Check sheet for the drawn part. Datum: minimum x, y, z corner. Units: mm. A direction names the side the tool comes from. Coordinates: 2 decimals unless noted, no trailing zeros. Loops run counter-clockwise (first coordinate to the right, second up) from the corner with the lowest first, then second, coordinate; pieces in that order, holes last. Notation, with made-up numbers: M -34.75,65.25 L 8.25,65.25 A30 cw 8.25,94.25 Z; hole C -12.5,-14 d4. An arc over 180 degrees is marked long. Answer in a Markdown table with one row per item. Add a question column.
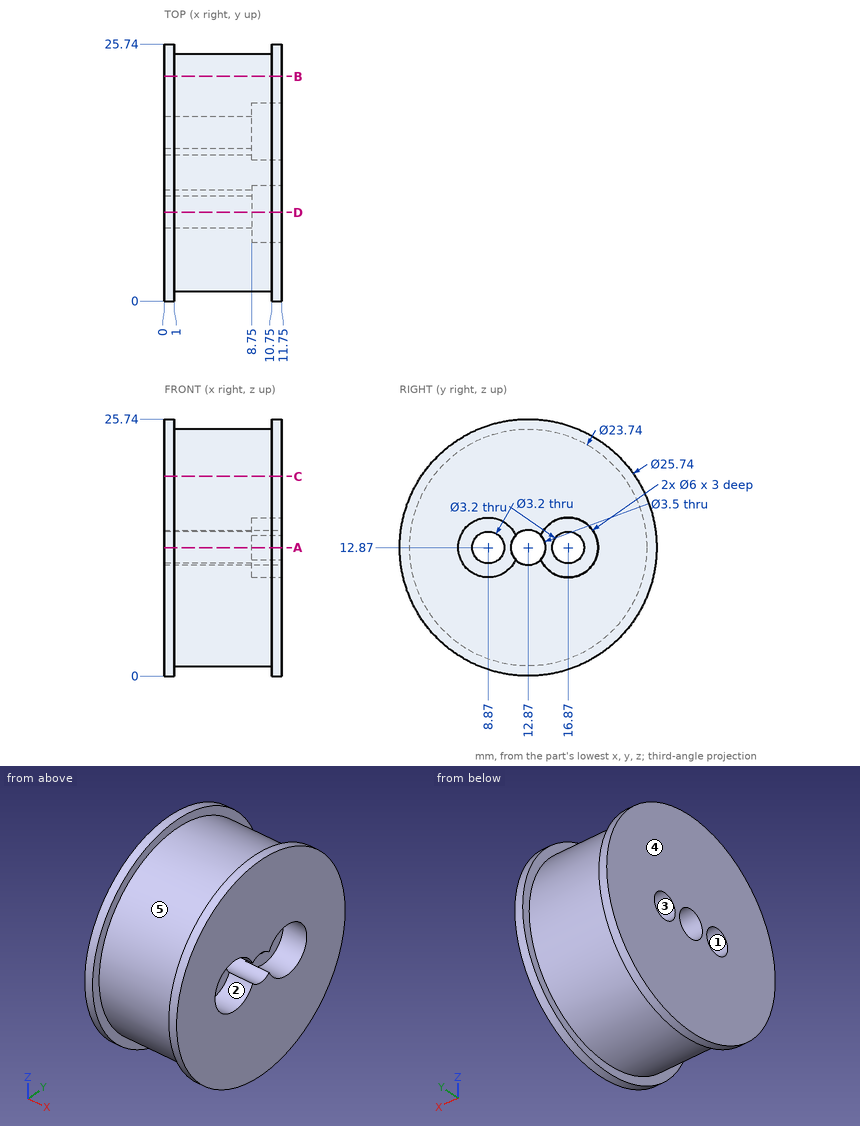
Q1. Access from +Z, -Z, +X, -X, +Y, -Y to the whole of each face (thin tool, end or side, straight path). Record for the marked faces 1 and 2.
Q2. Cross-section at B-B (y = 22.5). Record the cut outline in (x, z), plus the area to 3 significant figures.
Q3. Go/stop test with flat-tipped pins: pin 1 (4 mm diameter, centred on x = 4, y = 13.5, fed in from -Z); pin 2 (4 mm diameter, centred on x = 9, y = 11, fed in from +Z); pin 3 (1.7 mm diameter, centred on y = 9, z = 14, fed in from +X). Record where each tip stops, or that it passes through.
Q4. Cross-section at C-C (z = 20). Record the cut outline in (x, y).
Q5. Cross-section at D-D (y = 8.87). Record the cut outline in (x, z).
Q6. Mould release check, pull along Y, two halves, no side actions. Record for the marked faces 3, 4 and 5: released by +Y, released by -Y, zero draft, split by the parting line, or undercut.
Q7. Cross-section at A-A (z = 12.87). Record the cut outline in (x, y).
Q8. Thickness scan on L1, parallel to Y at x = 2.75, z = 12.87; L2, parallel to X at y = 2.25, z = 19.25; L3, parallel to Z at x = 1.75, y = 17. Record the ranges inside material, lowest first.
Answer key:
| question | item | result |
|---|---|---|
| 1 | face 1 | +X, -X |
| 1 | face 2 | +X |
| 2 | outline | M 0,4.33 L 1,4.33 L 1,5.93 L 10.75,5.93 L 10.75,4.33 L 11.75,4.33 L 11.75,21.41 L 10.75,21.41 L 10.75,19.81 L 1,19.81 L 1,21.41 L 0,21.41 Z |
| 2 | area | 169 mm^2 |
| 3 | pin 1 | z = 1 |
| 3 | pin 2 | z = 25.71 |
| 3 | pin 3 | x = 8.75 |
| 4 | outline | M 0,2.16 L 1,2.16 L 1,3.38 L 10.75,3.38 L 10.75,2.16 L 11.75,2.16 L 11.75,23.58 L 10.75,23.58 L 10.75,22.36 L 1,22.36 L 1,23.58 L 0,23.58 Z |
| 5 | outline | M 0,0.64 L 1,0.64 L 1,1.69 L 10.75,1.69 L 10.75,0.64 L 11.75,0.64 L 11.75,9.87 L 8.75,9.87 L 8.75,11.27 L 0,11.27 Z; M 0,14.47 L 8.75,14.47 L 8.75,15.87 L 11.75,15.87 L 11.75,25.1 L 10.75,25.1 L 10.75,24.05 L 1,24.05 L 1,25.1 L 0,25.1 Z |
| 6 | face 3 | undercut |
| 6 | face 4 | zero draft |
| 6 | face 5 | split by the parting line |
| 7 | outline | M 0,0 L 1,0 L 1,1 L 10.75,1 L 10.75,0 L 11.75,0 L 11.75,5.87 L 8.75,5.87 L 8.75,7.27 L 0,7.27 Z; M 0,10.47 L 8.75,10.47 L 8.75,11.12 L 0,11.12 Z; M 0,14.62 L 8.75,14.62 L 8.75,15.27 L 0,15.27 Z; M 0,18.47 L 8.75,18.47 L 8.75,19.87 L 11.75,19.87 L 11.75,25.74 L 10.75,25.74 L 10.75,24.74 L 1,24.74 L 1,25.74 L 0,25.74 Z |
| 8 | L1 | 1 to 7.27, 10.47 to 11.12, 14.62 to 15.27, 18.47 to 24.74 |
| 8 | L2 | 0 to 1, 10.75 to 11.75 |
| 8 | L3 | 1.74 to 11.28, 14.46 to 24 |
